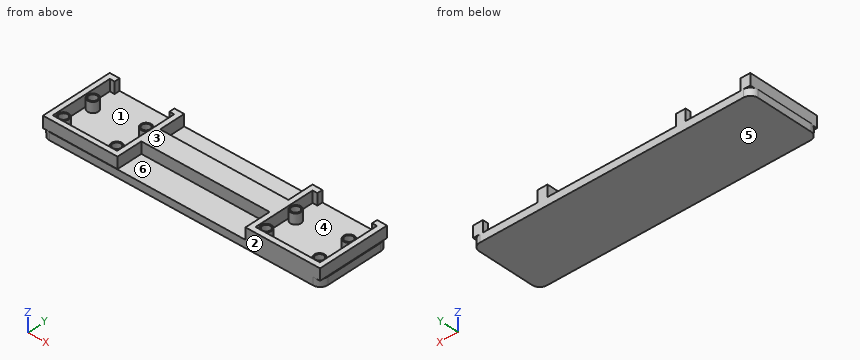
from build123d import *

# Parameters (mm, degrees)
SKETCH1_W                  = 110
SKETCH1_H                  = 28.5
BACKPLATE_BASE_DEPTH       = 3
OUTER_CORNER_FILLETS_R     = 3
SKETCH2_W                  = 29.4
SKETCH2_H                  = 28.381
SKETCH2_W_2                = 25.4
SKETCH2_H_2                = 24.262
SKETCH2_H_3                = 28.5
POCKET_WALLS_DEPTH         = 4.5
SKETCH3_W                  = 50.6
SKETCH3_H                  = 8
CENTER_BRIDGE_DEPTH        = 4.5
SKETCH4_W                  = 21.6
SKETCH4_H                  = 3
CSI_CABLE_EXIT_SLOTS_DEPTH = 4.5
STANDOFF_BOSSES_START      = 3
SKETCH5_R                  = 2.1
STANDOFF_BOSSES_DEPTH      = 4
SKETCH6_R                  = 1.6
M2_INSERT_HOLES_DEPTH      = 4.5


with BuildPart() as part:
    # Sketch1 → Backplate_Base (new body)
    with BuildSketch(Plane.XY):
        Rectangle(SKETCH1_W, SKETCH1_H)
    extrude(amount=BACKPLATE_BASE_DEPTH)

    # Outer_Corner_Fillets
    outer_corner_fillets_edges = [part.edges().sort_by_distance(p)[0] for p in [
        (-55, 14.25, 1.5),
        (55, 14.25, 1.5),
        (55, -14.25, 1.5),
        (-55, -14.25, 1.5),
    ]]
    fillet(outer_corner_fillets_edges, radius=OUTER_CORNER_FILLETS_R)

    # Sketch2 → Pocket_Walls (add)
    # profile 1 of 2: a face of its own
    with BuildSketch(Plane.XY.offset(3)):
        with Locations((-40, 0.0595)):
            Rectangle(SKETCH2_W, SKETCH2_H)
        with Locations((-40, 0)):
            Rectangle(SKETCH2_W_2, SKETCH2_H_2, mode=Mode.SUBTRACT)
    # profile 2 of 2: a face of its own
    with BuildSketch(Plane.XY.offset(3)):
        with Locations((40, 0)):
            Rectangle(SKETCH2_W, SKETCH2_H_3)
        with Locations((40, 0)):
            Rectangle(SKETCH2_W_2, SKETCH2_H_2, mode=Mode.SUBTRACT)
    extrude(amount=POCKET_WALLS_DEPTH)

    # Sketch3 → Center_Bridge (add)
    with BuildSketch(Plane.XY.offset(3)):
        Rectangle(SKETCH3_W, SKETCH3_H)
    extrude(amount=CENTER_BRIDGE_DEPTH)

    # Sketch4 → CSI_Cable_Exit_Slots (cut)
    with BuildSketch(Plane.XY.offset(7.5)):
        with Locations((-40, 13.131)):
            Rectangle(SKETCH4_W, SKETCH4_H)
        with Locations((40, 13.131)):
            Rectangle(SKETCH4_W, SKETCH4_H)
    extrude(amount=-CSI_CABLE_EXIT_SLOTS_DEPTH, mode=Mode.SUBTRACT)

    # Sketch5 → Standoff_Bosses (add)
    with BuildSketch(Plane.XY.offset(STANDOFF_BOSSES_START)):
        with Locations(Location((-50.5, -9.931, 0), (0, 0, 180))):
            Circle(SKETCH5_R)
        with Locations(Location((-29.5, -9.931, 0), (0, 0, 180))):
            Circle(SKETCH5_R)
        with Locations(Location((-50.5, 2.569, 0), (0, 0, 180))):
            Circle(SKETCH5_R)
        with Locations(Location((-29.5, 2.569, 0), (0, 0, 180))):
            Circle(SKETCH5_R)
        with Locations(Location((29.5, -9.931, 0), (0, 0, 180))):
            Circle(SKETCH5_R)
        with Locations(Location((50.5, -9.931, 0), (0, 0, 180))):
            Circle(SKETCH5_R)
        with Locations(Location((29.5, 2.569, 0), (0, 0, 180))):
            Circle(SKETCH5_R)
        with Locations(Location((50.5, 2.569, 0), (0, 0, 180))):
            Circle(SKETCH5_R)
    extrude(amount=STANDOFF_BOSSES_DEPTH)

    # Sketch6 → M2_Insert_Holes (cut)
    with BuildSketch(Plane.XY.offset(7)):
        with Locations((-50.5, -9.931)):
            Circle(SKETCH6_R)
        with Locations((-29.5, -9.931)):
            Circle(SKETCH6_R)
        with Locations((-50.5, 2.569)):
            Circle(SKETCH6_R)
        with Locations((-29.5, 2.569)):
            Circle(SKETCH6_R)
        with Locations((29.5, -9.931)):
            Circle(SKETCH6_R)
        with Locations((50.5, -9.931)):
            Circle(SKETCH6_R)
        with Locations((29.5, 2.569)):
            Circle(SKETCH6_R)
        with Locations((50.5, 2.569)):
            Circle(SKETCH6_R)
    extrude(amount=-M2_INSERT_HOLES_DEPTH, mode=Mode.SUBTRACT)


solid = part.part
CAD build for the part. Positions are in the model's coordinates, mm. Face numbers are marked on the shaded views. A direction names the side the tool comes from. Give positions to 0.01 mm unless a question says otherwise; leave off trailing zeros. Loops run counter-clockwise (first coordinate to the right, second up) from the corner with the lowest first, then second, coordinate; pieces in that order, holes last. Notation, with made-up numbers: M 61,23.25 L 101,23.25 A11 cw 101,40.25 Z; hole C -4,6.25 d5. An arc over 180 degrees is marked long. Answer in a Markdown table with one row per item. Add a question column.
Item 1: Band-saw the part on A-A on x = 4.5. Give the cut face in (y, z), then the cut area to 4 significant figures.
Item 2: Probe probe 1 along X at (y, z) = (-3.25, 5); probe 2 along X at (y, z) = (9.5, 6.25); probe 3 along Z at (x, y) = (-34, 1). List the from-to ranges inside material, lowest first.
Item 3: Band-saw the part on B-B on z = 4.75. Give the number of separate pieces and of enclosed holes in the cut face, then the cut area to 3 significant figures.
Item 4: Band-saw the part on D-D on x = 42. Give the cut face in (y, z).
Item 5: Drop flat-ended pins along their axis: P1, Ø1.5, axis at x = -7, z = 4.5, coming from the -Y side; P2, Ø2, axis at x = -12, z = 5.5, coming from the +Y side; P3, Ø2, axis at y = -4, z = 6.5, coming from the -X side. Give the stop position or say it passes through.
Item 6: Tool access for the marked faces 4, 5 and 6: list every direction of +Z, -Z, +X, -X, +Y, -Y with a clear straight run to the whole face (end or side of a thin tool).
Item 7: Band-saw the part on C-C on x = -41.5. Give the cut face in (y, z), then the cut area to 3 significant figures.
Item 8: Mould opens along Y. For the marked faces 1, 2 and 3 say: +Y half, -Y half, draft (parallel to the pull), parting line (faces both ways), or undercut.
Reply:
| question | item | result |
|---|---|---|
| 1 | outline | M -14.25,0 L 14.25,0 L 14.25,3 L 4,3 L 4,7.5 L -4,7.5 L -4,3 L -14.25,3 Z |
| 1 | area | 121.5 mm^2 |
| 2 | probe 1 | x = -54.7 to -52.7, -27.3 to 27.3, 52.7 to 54.7 |
| 2 | probe 2 | x = -54.7 to -52.7, -27.3 to -25.3, 25.3 to 27.3, 52.7 to 54.7 |
| 2 | probe 3 | z = 0 to 3 |
| 3 | separate pieces | 9 |
| 3 | enclosed holes | 8 |
| 3 | area | 800 mm^2 |
| 4 | outline | M -14.25,0 L 14.25,0 L 14.25,3 L -12.13,3 L -12.13,7.5 L -14.25,7.5 Z |
| 5 | P1 | stops at y = -4 |
| 5 | P2 | stops at y = 4 |
| 5 | P3 | stops at x = -54.7 |
| 6 | face 4 | +Z |
| 6 | face 5 | -Z, +X, -X, +Y, -Y |
| 6 | face 6 | +Z, -Y |
| 7 | outline | M -14.25,0 L 14.25,0 L 14.25,3 L -12.13,3 L -12.13,7.5 L -14.13,7.5 L -14.13,3 L -14.25,3 Z |
| 7 | area | 94.5 mm^2 |
| 8 | face 1 | undercut |
| 8 | face 2 | -Y half |
| 8 | face 3 | draft |
